from build123d import *

# Parameters (mm, degrees)
SKETCH1_R           = 1.5
SKETCH1_R_2         = 1
SKETCH1_R_3         = 7
SKETCH1_R_4         = 4.75
BOSS_EXTRUDE1_DEPTH = 3


with BuildPart() as part:
    # Sketch1 → Boss-Extrude1 (new body)
    with BuildSketch(Plane(origin=(0, 0, 0), x_dir=(0, 0, -1), z_dir=(1, 0, 0))):
        with BuildLine():
            Line((-48.375, 0), (48.375, 0))
            ThreePointArc((48.375, 0), (67.125, 18.75), (48.375, 37.5))
            Line((48.375, 37.5), (40.375, 37.5))
            ThreePointArc((40.375, 37.5), (35.295765254, 38.742880835), (31.364327513, 42.1906592))
            ThreePointArc((31.364327513, 42.1906592), (-27.467628368, 101.587088748), (-102.722095146, 138))
            ThreePointArc((-102.722095146, 138), (-113.291936406, 127.38864025), (-103.88918697, 115.730561375))
            ThreePointArc((-103.88918697, 115.730561375), (-50.193524878, 91.468412174), (-15.975, 43.5))
            ThreePointArc((-15.975, 43.5), (-20.221951673, 33.246951673), (-30.475, 29))
            Line((-30.475, 29), (-48.375, 29))
            ThreePointArc((-48.375, 29), (-62.875, 14.5), (-48.375, 0))
        make_face()
        with Locations((59.625, 18.75)):
            Circle(SKETCH1_R, mode=Mode.SUBTRACT)
        with Locations((54.625, 28.75)):
            Circle(SKETCH1_R_2, mode=Mode.SUBTRACT)
        with Locations((-47.875, 14.5)):
            Circle(SKETCH1_R_3, mode=Mode.SUBTRACT)
        with Locations((-103.305641058, 126.865280687)):
            Circle(SKETCH1_R_4, mode=Mode.SUBTRACT)
        with BuildLine():
            Line((46.625, 23.25), (48.625, 23.25))
            ThreePointArc((48.625, 23.25), (53.125, 18.75), (48.625, 14.25))
            Line((48.625, 14.25), (46.625, 14.25))
            ThreePointArc((46.625, 14.25), (42.125, 18.75), (46.625, 23.25))
        make_face(mode=Mode.SUBTRACT)
        with BuildLine():
            Line((-84.112179989, 120.210043762), (-78.004177954, 117.98691283))
            ThreePointArc((-78.004177954, 117.98691283), (-76.659414879, 115.103059111), (-79.543268599, 113.758296037))
            Line((-79.543268599, 113.758296037), (-85.651270634, 115.981426968))
            ThreePointArc((-85.651270634, 115.981426968), (-86.996033708, 118.865280687), (-84.112179989, 120.210043762))
        make_face(mode=Mode.SUBTRACT)
        with BuildLine():
            Line((-75.120324234, 124.438660555), (-69.012322199, 122.215529624))
            ThreePointArc((-69.012322199, 122.215529624), (-67.667559125, 119.331675904), (-70.551412844, 117.98691283))
            Line((-70.551412844, 117.98691283), (-76.659414879, 120.210043762))
            ThreePointArc((-76.659414879, 120.210043762), (-78.004177954, 123.093897481), (-75.120324234, 124.438660555))
        make_face(mode=Mode.SUBTRACT)
    extrude(amount=BOSS_EXTRUDE1_DEPTH)


solid = part.part
Input: part model. Units: mm. Frame: model coordinates. A direction names the side the tool comes from. Give positions to 0.01 mm unless a question says otherwise; leave off trailing zeros. Order: outer loops, then holes, each group sorted by start corner. A loop starts at its lowest first (then second) coordinate and runs counter-clockwise, first axis right, second up. Notation, with made-up numbers: (62.5, 26.25) -> (94.5, 26.25) arc R26 cw to (94.5, 63.25) -> close; hole circle Ø6 at (42.25, 75). An arc over 180 degrees is marked (long way). Use one line per item in the form item = value.
1) Mould query, pull axis Z, two halves, no side actions, for faces 4 (the cylindrical face through (1.479, 127.618, 113.278)), 5 (the cylindrical face through (1.48, 38.71, -35.36)), 6 (the cylindrical face through (1.479, 18.849, -53.124)). Classes: pulls with the +Z half, pulls with the -Z half, needs draft (parallel to the pull), parting line crosses it, or undercut.
Response values:
face_4 = pulls with the +Z half
face_5 = pulls with the -Z half
face_6 = undercut
2) Section A-A, the plane z = 44.5. Return loops of the section in (x, y), and give its area (3 significant figures).
Response values:
outline = (0, 0) -> (3, 0) -> (3, 8.37) -> (0, 8.37) -> close; (0, 20.63) -> (3, 20.63) -> (3, 29) -> (0, 29) -> close; (0, 86.46) -> (3, 86.46) -> (3, 112.73) -> (0, 112.73) -> close
area = 129 mm^2
3) First-contact query: pin 1 Ø0.9 at (x, z) = (2, 40) entering from +Y; pin 2 Ø1.5 at (x, z) = (1, -45) entering from +Y; pin 3 Ø8.5 at (y, z) = (14.5, 47.875) entering from +X; pin 4 Ø1.5 at (x, z) = (2.5, -31) entering from +Y. Flat tips, straight axial feed; report the tip coordinate or a pass-through.
Response values:
pin_1 = 110.26
pin_2 = 37.5
pin_3 = through
pin_4 = 43.77
4) Section D-D, the plane z = -37.5. Return loops of the section in (x, y), and give its area (3 significant figures).
Response values:
outline = (0, 0) -> (3, 0) -> (3, 37.88) -> (0, 37.88) -> close
area = 114 mm^2
5) Reachability of faces 1 (the flat face through (0, 49, 10)), 2 (the cylindrical face through (1.479, 18.651, -42.126)), 3 (the cylindrical face through (1.479, 91.996, 50.84)) from +Z, -Z, +X, -X, +Y, -Y: full face, straight path, thin tool, end or side. Return the list, or none.
Response values:
face_1 = +Z, -Z, -X, +Y, -Y
face_2 = +X, -X
face_3 = +Z, +X, -X
6) Section B-B, the plane x = 1. Return loops of the section in (y, z) (3 decimals), and give its area (3 significant figures).
Response values:
outline = (0, -48.375) arc R18.75 ccw to (37.5, -48.375) -> (37.5, -40.375) arc R11 cw to (42.191, -31.364) arc R247.422 ccw to (138, 102.722) arc R11.216 ccw to (115.731, 103.889) arc R113.159 cw to (43.5, 15.975) arc R14.5 cw to (29, 30.475) -> (29, 48.375) arc R14.5 ccw to (0, 48.375) -> close; hole circle Ø14 at (14.5, 47.875); hole (14.25, -48.625) arc R4.5 ccw to (23.25, -48.625) -> (23.25, -46.625) arc R4.5 ccw to (14.25, -46.625) -> close; hole circle Ø3 at (18.75, -59.625); hole circle Ø2 at (28.75, -54.625); hole (113.758, 79.543) arc R2.25 ccw to (117.987, 78.004) -> (120.21, 84.112) arc R2.25 ccw to (115.981, 85.651) -> close; hole (117.987, 70.551) arc R2.25 ccw to (122.216, 69.012) -> (124.439, 75.12) arc R2.25 ccw to (120.21, 76.659) -> close; hole circle Ø9.5 at (126.865, 103.306)
area = 7,890 mm^2
7) Line query: probe 1 along Y at (x, z) = (1.3, -46.5); probe 2 along Y at (x, z) = (1.9, 86); probe 3 along Y at (x, z) = (0.9, 48). Output: solid intervals per line, ascending.
Response values:
probe_1 = 0 to 14.25, 23.25 to 37.5
probe_2 = 111.31 to 116.14, 120.05 to 132.52
probe_3 = 0 to 7.5, 21.5 to 29, 89.62 to 114.78
8) Section C-C, the plane z = -11. Return loops of the section in (x, y).
Response values:
outline = (0, 0) -> (3, 0) -> (3, 67.55) -> (0, 67.55) -> close
